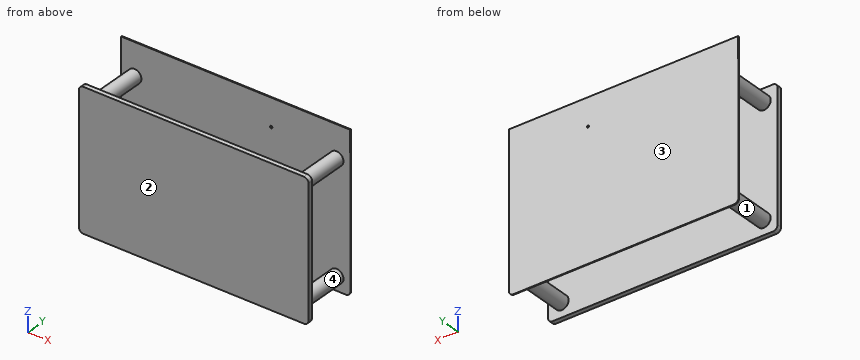
from build123d import *

# Parameters (mm, degrees)
BOSS_EXTRUDE1_DEPTH = 10
SKETCH2_R           = 15
BOSS_EXTRUDE2_DEPTH = 109
BOSS_EXTRUDE3_DEPTH = 2
SKETCH4_W           = 498.700760334
SKETCH4_H           = 80
BOSS_EXTRUDE4_DEPTH = 2
SKETCH5_R           = 2.5
CUT_EXTRUDE1_DEPTH  = 20


with BuildPart() as part:
    # Sketch1 → Boss-Extrude1 (new body)
    with BuildSketch(Plane(origin=(0, 0, 0), x_dir=(1, 0, 0), z_dir=(0, 1, 0))):
        with BuildLine():
            Line((-240, 150), (240, 150))
            ThreePointArc((240, 150), (247.071067812, 147.071067812), (250, 140))
            Line((250, 140), (250, -140))
            ThreePointArc((250, -140), (247.071067812, -147.071067812), (240, -150))
            Line((240, -150), (-240, -150))
            ThreePointArc((-240, -150), (-247.071067812, -147.071067812), (-250, -140))
            Line((-250, -140), (-250, 140))
            ThreePointArc((-250, 140), (-247.071067812, 147.071067812), (-240, 150))
        make_face()
    extrude(amount=BOSS_EXTRUDE1_DEPTH)

    # Sketch2 → Boss-Extrude2 (add)
    with BuildSketch(Plane(origin=(0, 10, 0), x_dir=(1, 0, 0), z_dir=(0, 1, 0))):
        with Locations(Location((-220, 120, 0), (0, 0, 90))):
            Circle(SKETCH2_R)
        with Locations(Location((220, 120, 0), (0, 0, 90))):
            Circle(SKETCH2_R)
        with Locations(Location((220, -120, 0), (0, 0, 90))):
            Circle(SKETCH2_R)
        with Locations(Location((-220, -120, 0), (0, 0, 90))):
            Circle(SKETCH2_R)
    extrude(amount=BOSS_EXTRUDE2_DEPTH)

    # Sketch3 → Boss-Extrude3 (add)
    with BuildSketch(Plane(origin=(0, 119, 0), x_dir=(1, 0, 0), z_dir=(0, 1, 0))):
        with BuildLine():
            Line((-240, 150), (240, 150))
            ThreePointArc((240, 150), (247.071067812, 147.071067812), (250, 140))
            Line((250, 140), (250, -140))
            ThreePointArc((250, -140), (247.071067812, -147.071067812), (240, -150))
            Line((240, -150), (-240, -150))
            ThreePointArc((-240, -150), (-247.071067812, -147.071067812), (-250, -140))
            Line((-250, -140), (-250, 140))
            ThreePointArc((-250, 140), (-247.071067812, 147.071067812), (-240, 150))
        make_face()
    extrude(amount=BOSS_EXTRUDE3_DEPTH)

    # Sketch4 → Boss-Extrude4 (add)
    with BuildSketch(Plane(origin=(0, 121, 0), x_dir=(1, 0, 0), z_dir=(0, 1, 0))):
        with Locations((0, -150)):
            Rectangle(SKETCH4_W, SKETCH4_H)
    extrude(amount=-BOSS_EXTRUDE4_DEPTH)

    # Sketch5 → Cut-Extrude1 (cut)
    with BuildSketch(Plane(origin=(0, 121, 0), x_dir=(1, 0, 0), z_dir=(0, 1, 0))):
        with Locations(Location((77.630380167, -130, 0), (0, 0, 270))):
            Circle(SKETCH5_R)
    extrude(amount=-CUT_EXTRUDE1_DEPTH, mode=Mode.SUBTRACT)


solid = part.part
Could you check a few things on this model? Use its own coordinates, in mm. Face numbers are marked on the shaded views. A direction names the side the tool comes from. Coordinates: 2 decimals unless noted, no trailing zeros. Loops run counter-clockwise (first coordinate to the right, second up) from the corner with the lowest first, then second, coordinate; pieces in that order, holes last.
1. Imagine slicing it at D-D (x = -220). Please give me the cut outline in (y, z), and give its area (3 significant figures).
2. Imagine slicing it at A-A (z = -83). Please give me the cut outline in (x, y), and give its area (3 significant figures).
3. Imagine slicing it at C-C (z = 120). Please give me the cut outline in (x, y).
4. For the marked faces 1 and 2, which set-ups out of +Z, -Z, +X, -X, +Y, -Y let a thin tool reach every point of the face, with its end or its side?
5. We'd pull the mould along X, two halves only. Please class the marked faces 3 and 4: released by +X, released by -X, zero draft, split by the parting line, or undercut.
6. For P1, Ø0.6, axis at y = 119.5, z = 156, coming from the +X side; P2, Ø12, axis at y = 15.5, z = -80.5, coming from the +X side; P3, Ø3, axis at x = 12, y = 5.5, coming from the +Z side; P4, Ø8, axis at y = 18.5, z = 114.5, coming from the +X side, each with a flat end and sliding along its axis, tell me the tip position at first contact or that it passes through.
7. Imagine slicing it at B-B (x = -34.5). Please give me the cut outline in (y, z), and give its area (3 significant figures).
8. I need wall thicknesses on L1, parallel to Y at x = 93, z = -10.5; L2, parallel to X at y = 120.05, z = 130; L3, parallel to X at y = 110, z = -119. Which ranges of each line are inside material? Lowest first, please.
Computed values:
1. outline: (0, -150) - (10, -150) - (10, -135) - (119, -135) - (119, -150) - (121, -150) - (121, 190) - (119, 190) - (119, 135) - (10, 135) - (10, 150) - (0, 150) - close; hole (10, -105) - (119, -105) - (119, 105) - (10, 105) - close
1. area: 10,200 mm2
2. outline: (-250, 0) - (250, 0) - (250, 10) - (-250, 10) - close; (-250, 119) - (250, 119) - (250, 121) - (-250, 121) - close
2. area: 6,000 mm2
3. outline: (-250, 0) - (250, 0) - (250, 10) - (235, 10) - (235, 119) - (250, 119) - (250, 121) - (-250, 121) - (-250, 119) - (-235, 119) - (-235, 10) - (-250, 10) - close; hole (-205, 10) - (205, 10) - (205, 119) - (-205, 119) - close
4. face 1: none
4. face 2: +Z, -Z, +X, -X, -Y
5. face 3: zero draft
5. face 4: undercut
6. P1: stops at x = 249.35
6. P2: stops at x = 250
6. P3: stops at z = 150
6. P4: stops at x = 234.92
7. outline: (0, -150) - (10, -150) - (10, 150) - (0, 150) - close; (119, -150) - (121, -150) - (121, 190) - (119, 190) - close
7. area: 3,680 mm2
8. L1: y = 0 to 10, 119 to 121
8. L2: x = -250 to 75.13, 80.13 to 250
8. L3: x = -234.97 to -205.03, 205.03 to 234.97
